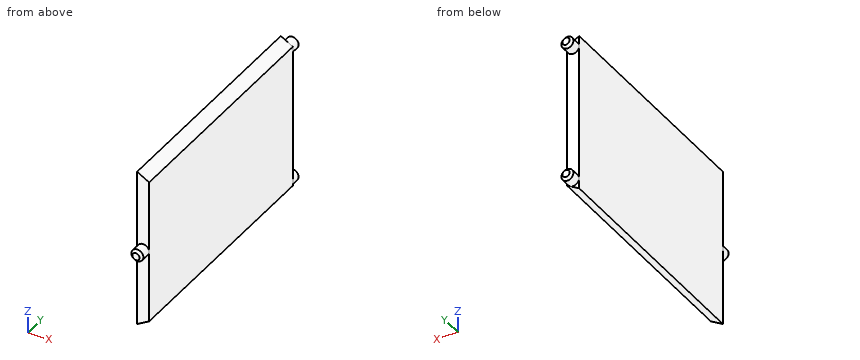
Autodesk Inventor part; units mm, degrees
ref_plane "YZ Plane" through (0, 0, 0) normal (1, 0, 0) x (0, 1, 0)
ref_plane "XZ Plane" through (0, 0, 0) normal (0, 1, 0) x (-1, 0, 0)
ref_plane "XY Plane" through (0, 0, 0) normal (0, 0, 1) x (1, 0, 0)
sketch "스케치2" plane through (0, 0, 0) normal (0, 1, 0) x (-1, 0, 0)
  line L0 (0, -60) -> (-51.9615, -30)
  line L1 (-51.9615, -30) -> (-51.9615, 30)
  line L2 (-51.9615, 30) -> (0, 60)
  line L3 (0, 60) -> (51.9615, 30)
  line L4 (51.9615, 30) -> (51.9615, -30)
  line L5 (51.9615, -30) -> (0, -60)
  line L6 (0, -65.7735) -> (-56.9615, -32.8868)
  line L7 (-56.9615, -32.8868) -> (-56.9615, 32.8868)
  line L8 (-56.9615, 32.8868) -> (0, 65.7735)
  line L9 (0, 65.7735) -> (56.9615, 32.8868)
  line L10 (56.9615, 32.8868) -> (56.9615, -32.8868)
  line L11 (56.9615, -32.8868) -> (0, -65.7735)
  line L12 (51.9615, -30) -> (56.9615, -32.8868)
  line L13 (56.9615, 32.8868) -> (51.9615, 30)
  point P0 (0, 0)
  point P1 (0, 0)
  dimension "d0" = 60
  dimension "d1" = 5
extrude "돌출1" add sketch "스케치2" along normal blind 100 contours L4 L13 L10 L12
sketch "스케치3" plane through (0, 100, 0) normal (0, 1, 0) x (1, 0, 0)
  line L0 (-56.9615, -32.8868) -> (-51.9615, -30) construction
  line L1 (-51.9615, 30) -> (-56.9615, 32.8868) construction
  line L2 (-56.9615, 32.8868) -> (-56.9615, -32.8868) construction
  circle A0 centre (-54.4615, 28.5566) radius 2.5
  circle A1 centre (-54.4615, -28.5566) radius 2.5
  point P0 (0, 0)
  dimension "d4" = 5
  dimension "d5" = 5
extrude "돌출2" add sketch "스케치3" along normal blind 5
sketch "스케치4" plane through (0, 0, 0) normal (0, -1, 0) x (1, 0, 0)
  line L0 (-51.9615, 30) -> (-51.9615, -30) construction
  circle A0 centre (-54.4615, 0) radius 2.5
  point P0 (0, 0)
  dimension "d8" = 5
extrude "돌출3" add sketch "스케치4" along normal blind 5
chamfer "모따기1" distance 1 angle 45 3 edges at (-56.9615, 105, 28.5566) (-56.9615, 105, -28.5566) (-56.9615, -5, 0)
properties part number "col"
Verification items for the finished model (mm, model axes). Round coordinates to 2 decimals unless told otherwise and drop trailing zeros. Loops run counter-clockwise (first coordinate to the right, second up) from the corner with the lowest first, then second, coordinate; pieces in that order, holes last. Notation, with made-up numbers: (52, 61) - (100, 61) arc R12 cw to (100, 70) - close; hole circle Ø8 at (74.25, 82.25). An arc over 180 degrees is marked (long way). Answer in a Markdown table with one row per item. Add a question column.
Q1. Section check A-A on y = 70. Enter the section's corners in (x, z).
Q2. Section check B-B on z = 10. Enter the section's corners in (x, y).
Q3. Gauge pin test, flat ends, axial feed: pin 1 (2.5 mm diameter, centred on x = -53.5, z = 24.5, fed in from -Y); pin 2 (1.5 mm diameter, centred on x = -54.5, z = -5.5, fed in from +Y). Record the tip position at first contact, or that the pin passes through.
Q4. Material ranges on line 1 (Y direction, x = -54.3, z = -6.5); line 2 (Y direction, x = -52.8, z = -1); line 3 (Z direction, x = -55.65, y = 84), recorded low to high.
Found:
| question | item | result |
|---|---|---|
| 1 | outline | (-56.96, -32.89) - (-51.96, -30) - (-51.96, 30) - (-56.96, 32.89) - close |
| 2 | outline | (-56.96, 0) - (-51.96, 0) - (-51.96, 100) - (-56.96, 100) - close |
| 3 | pin 1 | stops at y = 0 |
| 3 | pin 2 | stops at y = 100 |
| 4 | line 1 | y = 0 to 100 |
| 4 | line 2 | y = -4.56 to 100 |
| 4 | line 3 | z = -32.13 to 32.13 |
